Check sheet for the modelled part. Datum: model origin and axes. Units: mm. Face numbers are marked on the shaded views. A direction names the side the tool comes from. Coordinates: 2 decimals unless noted, no trailing zeros. Write each loop counter-clockwise with the first axis right and the second up, starting at its lowest first coordinate (ties: lowest second). Pieces come first, ordered by that corner, then holes. Notation, with made-up numbers: M 42.5,18 L 89.5,18 A21 ccw 89.5,42 Z; hole C -31.5,-36 d4. An arc over 180 degrees is marked long. Answer as CSV lines item,"result". Start each with the question number.
Q1. Sectioned sample at B-B, the plane x = -42. Record the cut outline in (y, z).
Q2. Depth check by flat-ended pin: pin 1 Ø8 at (y, z) = (-37.5, -25) entering from +X; pin 2 Ø0.8 at (x, z) = (64.5, -28) entering from +Y; pin 3 Ø10 at (x, y) = (5.5, 29) entering from -Z; pin 4 Ø7.5 at (y, z) = (-62.5, -20) entering from +X. Enter the tip coordinate at first touch or a pass-through.
Q3. Mould release check, pull along Y, two halves, no side actions. Record for the marked faces 1, 2 and 3: pulls with the +Y half, pulls with the -Y half, needs draft (parallel to the pull), parting line crosses it, or undercut.
Q4. Sectioned sample at A-A, the plane z = -6. Count the separate pieces of the cut face and the enclosed holes in it, then the cut area to 3 significant figures.
Q5. Sectioned sample at C-C, the plane y = 25. Record the cut outline in (x, z), then the cut area to 3 significant figures.
Q6. Thickness scan on line 1 along Y through (x, z) = (55.5, -24.5). Record the ranges inside material, lowest first. Write a range as from..to.
Q7. Access from +Z, -Z, +X, -X, +Y, -Y to the whole of each face (thin tool, end or side, straight path). Record for the marked faces 4, 5 and 6.
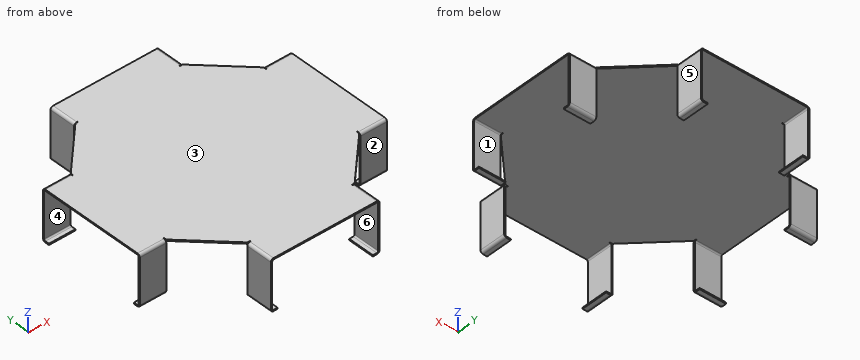
from build123d import *

# Parameters (mm, degrees)
SM_BASE_FLANGE_1_DEPTH            = 0.75
SM_EDGE_FLANGE_1_STRIP_W          = 4.5
SM_EDGE_FLANGE_1_STRIP_H          = 0.75
SM_EDGE_FLANGE_1_STRIP_CUT_DEPTH  = 15
SM_EDGE_FLANGE_1_RELIEF_W         = 4.875
SM_EDGE_FLANGE_1_RELIEF_H         = 0.375
SM_EDGE_FLANGE_1_RELIEF_CUT_DEPTH = 0.75
SM_EDGE_FLANGE_1_DEPTH            = 15
SM_EDGE_FLANGE_2_STRIP_W          = 4.5
SM_EDGE_FLANGE_2_STRIP_H          = 0.75
SM_EDGE_FLANGE_2_STRIP_CUT_DEPTH  = 15
SM_EDGE_FLANGE_2_DEPTH            = 15


# Sheet-metal steps are written as plain solids
with BuildPart() as part:
    # Sketch 1 → Базовая кромка1 (new body)
    with BuildSketch(Plane.XY):
        Polygon((-70, 0), (-70, 30), (-55, 30), (-42.5, 42.5), (0, 0), align=None)
    extrude(amount=-SM_BASE_FLANGE_1_DEPTH)

    # Ребро-кромка1 strip (across the edge) → Ребро-кромка1 strip cut (cut)
    with BuildSketch(Plane(origin=(-70, 30, -0.75), x_dir=(0, -1, 0), z_dir=(1, 0, 0))):
        with Locations((-1.5, -0.375)):
            Rectangle(SM_EDGE_FLANGE_1_STRIP_W, SM_EDGE_FLANGE_1_STRIP_H)
    extrude(amount=SM_EDGE_FLANGE_1_STRIP_CUT_DEPTH, mode=Mode.SUBTRACT)

    # Ребро-кромка1 relief (on the sheet) → Ребро-кромка1 relief cut (cut)
    with BuildSketch(Plane(origin=(-70, 29.25, -0.75), x_dir=(0, -1, 0), z_dir=(0, 0, -1))):
        with Locations((-2.0625, -15.1875)):
            Rectangle(SM_EDGE_FLANGE_1_RELIEF_W, SM_EDGE_FLANGE_1_RELIEF_H)
    extrude(amount=-SM_EDGE_FLANGE_1_RELIEF_CUT_DEPTH, mode=Mode.SUBTRACT)

    # Ребро-кромка1 section (across the edge) → Ребро-кромка1 (add)
    with BuildSketch(Plane(origin=(-70, 30, -0.75), x_dir=(0, -1, 0), z_dir=(1, 0, 0))):
        with BuildLine():
            Line((-0.75, 0.75), (-0.75, 27))
            Line((-0.75, 27), (0, 27))
            Line((0, 27), (0, 0.75))
            ThreePointArc((0, 0.75), (0.219669914, 0.219669914), (0.75, 0))
            Line((0.75, 0), (0.75, -0.75))
            ThreePointArc((0.75, -0.75), (-0.310660172, -0.310660172), (-0.75, 0.75))
        make_face()
    extrude(amount=SM_EDGE_FLANGE_1_DEPTH)

    # Ребро-кромка2 strip (across the edge) → Ребро-кромка2 strip cut (cut)
    with BuildSketch(Plane(origin=(-70, 30, -27.75), x_dir=(0, 0, 1), z_dir=(1, 0, 0))):
        with Locations((-1.5, -0.375)):
            Rectangle(SM_EDGE_FLANGE_2_STRIP_W, SM_EDGE_FLANGE_2_STRIP_H)
    extrude(amount=SM_EDGE_FLANGE_2_STRIP_CUT_DEPTH, mode=Mode.SUBTRACT)

    # Ребро-кромка2 section (across the edge) → Ребро-кромка2 (add)
    with BuildSketch(Plane(origin=(-70, 30, -27.75), x_dir=(0, 0, 1), z_dir=(1, 0, 0))):
        with BuildLine():
            Line((-0.75, 0.75), (-0.75, 3))
            Line((-0.75, 3), (0, 3))
            Line((0, 3), (0, 0.75))
            ThreePointArc((0, 0.75), (0.219669914, 0.219669914), (0.75, 0))
            Line((0.75, 0), (0.75, -0.75))
            ThreePointArc((0.75, -0.75), (-0.310660172, -0.310660172), (-0.75, 0.75))
        make_face()
    extrude(amount=SM_EDGE_FLANGE_2_DEPTH)

    # Зеркальное отражение1: part across plane


with BuildPart() as part_1:
    add(part.part)
    add(part.part.mirror(Plane(origin=(-70, 0, -0.75), x_dir=(0, 0, 1), z_dir=(0, -1, 0))))

    # Зеркальное отражение2: part across plane


with BuildPart() as part_2:
    add(part_1.part)
    add(part_1.part.mirror(Plane(origin=(0, 0, -0.75), x_dir=(0, 0, 1), z_dir=(0.707106781186558, -0.7071067811865371, 0))))

    # Зеркальное отражение3: part across face


with BuildPart() as part_3:
    add(part_2.part)
    add(part_2.part.mirror(Plane(origin=(0, 0, -0.375), x_dir=(0, 0, 1), z_dir=(0.7071067811865476, 0.7071067811865476, 0))))


solid = part_3.part
Output:
1,outline,"M -43,-0.75 L 43,-0.75 L 43,0 L -43,0 Z"
2,pin 1,"passes through"
2,pin 2,"stops at y = 30.62"
2,pin 3,"stops at z = -0.75"
2,pin 4,"stops at x = 30.75"
3,face 1,"undercut"
3,face 2,"pulls with the -Y half"
3,face 3,"needs draft"
4,separate pieces,"8"
4,enclosed holes,"0"
4,area,"90.0 mm^2"
5,outline,"M -70,-0.75 L 70,-0.75 L 70,0 L -70,0 Z"
5,area,"105 mm^2"
6,line 1,"y = -30.75..-30, 30..30.75"
7,face 4,"+X, -X"
7,face 5,"+Z, -Z, +X, +Y, -Y"
7,face 6,"+Y, -Y"
